Can you work these out from the model? Positions are in its coordinate system, mm. A direction names the side the tool comes from. Give positions to 0.01 mm unless a question says otherwise; leave off trailing zeros. Loops run counter-clockwise (first coordinate to the right, second up) from the corner with the lowest first, then second, coordinate; pieces in that order, holes last. Notation, with made-up numbers: (13.5, 30.25) - (50.5, 30.25) arc R23 ccw to (50.5, 63.25) - close; hole circle Ø5 at (0, -11). An arc over 180 degrees is marked (long way). Answer as a JSON object with one key per item and string values.
```python
from build123d import *

# Parameters (mm, degrees)
SKETCH1_R           = 17.5
SKETCH1_R_2         = 15
BOSS_EXTRUDE1_DEPTH = 10
SKETCH2_R           = 37.5
SKETCH2_R_2         = 27.5
BOSS_EXTRUDE2_DEPTH = 10


with BuildPart() as part:
    # Sketch1 → Boss-Extrude1 (new body)
    with BuildSketch(Plane(origin=(0, 0, 0), x_dir=(0, 0, -1), z_dir=(1, 0, 0))):
        with BuildLine():
            ThreePointArc((30.555677848, -21.739377894), (0, 37.5), (-30.555677848, -21.739377894))
            ThreePointArc((-30.555677848, -21.739377894), (-10, -78.973363491), (-22.221723794, -138.545961778))
            ThreePointArc((-22.221723794, -138.545961778), (0, -175), (22.221723794, -138.545961778))
            ThreePointArc((22.221723794, -138.545961778), (10, -78.973363491), (30.555677848, -21.739377894))
        make_face()
        Circle(SKETCH1_R, mode=Mode.SUBTRACT)
        with Locations((0, -150)):
            Circle(SKETCH1_R_2, mode=Mode.SUBTRACT)
    extrude(amount=BOSS_EXTRUDE1_DEPTH)

    # Sketch2 → Boss-Extrude2 (add)
    with BuildSketch(Plane.ZY):
        Circle(SKETCH2_R)
        Circle(SKETCH2_R_2, mode=Mode.SUBTRACT)
    extrude(amount=BOSS_EXTRUDE2_DEPTH)


solid = part.part
```
1) Imagine slicing it at C-C on y = -150. Write out the boundary of the cut face in (x, z), and give its area (3 significant figures).
Check sheet entries:
{"outline": "(0, -25) - (10, -25) - (10, -15) - (0, -15) - close; (0, 15) - (10, 15) - (10, 25) - (0, 25) - close", "area": "200 mm2"}
2) Imagine slicing it at D-D on x = 6.5. Write out the boundary of the cut face in (y, z).
Check sheet entries:
{"outline": "(-138.55, -22.22) arc R112.54 cw to (-21.74, -30.56) arc R37.5 ccw (long way) to (-21.74, 30.56) arc R112.54 cw to (-138.55, 22.22) arc R25 ccw (long way) to start; hole circle Ø30 at (-150, 0); hole circle Ø35 at (0, 0)"}
3) Which directions (+Z, -Z, +X, -X, +Y, -Y) give clear straight access to the entire face, cutting with the end or side of a thin tool? Please do faces 5 (the cylindrical face through (-4.93, -26.846, -5.961)), 6 (the cylindrical face through (4.93, -79.834, -9.942)).
Check sheet entries:
{"face 5": "-X", "face 6": "-Z, +X, -X"}
4) Imagine slicing it at A-A on y = 0. Write out the boundary of the cut face in (x, z).
Check sheet entries:
{"outline": "(-10, -37.5) - (10, -37.5) - (10, -17.5) - (0, -17.5) - (0, -27.5) - (-10, -27.5) - close; (-10, 27.5) - (0, 27.5) - (0, 17.5) - (10, 17.5) - (10, 37.5) - (-10, 37.5) - close"}
5) I'm going to push flat-ended pins straight in: P1, Ø6, axis at y = -64.5, z = -16.5, coming from the -X side; P2, Ø16.5, axis at y = 11.5, z = -3, coming from the -X side; P3, Ø4, axis at x = -4, z = 26.5, coming from the +Y side; P4, Ø6, axis at x = 4.5, y = -152, coming from the -Z side. Where does each tip first touch, or does it pass through?
Check sheet entries:
{"P1": "through", "P2": "x = 0", "P3": "y = 28.39", "P4": "z = -25"}
6) If we mould it in two halves opening along Z, with no side actions, what happens to faces 1 (the cylindrical face through (4.93, -78.114, 10.065)), 2 (the cylindrical face through (4.93, -163.31, -6.92)), 3 (the cylindrical face through (4.93, -174.99, 0.72)), 4 (the flat face through (-10, 20, -20))? For each: released by +Z, released by -Z, zero draft, split by the parting line, or undercut.
Check sheet entries:
{"face 1": "released by +Z", "face 2": "undercut", "face 3": "split by the parting line", "face 4": "zero draft"}
7) I need wall thicknesses on L1, parallel to Y at x = 5.25, z = 0; L2, parallel to X at y = 18, z = 18; L3, parallel to Y at x = -2.75, z = 0. Which ranges of each line are inside material? Lowest first, please.
Check sheet entries:
{"L1": "-175 to -165, -135 to -17.5, 17.5 to 37.5", "L2": "0 to 10", "L3": "-37.5 to -27.5, 27.5 to 37.5"}
8) Imagine slicing it at B-B on z = 0. Write out the boundary of the cut face in (x, y).
Check sheet entries:
{"outline": "(-10, -37.5) - (0, -37.5) - (0, -135) - (10, -135) - (10, -17.5) - (0, -17.5) - (0, -27.5) - (-10, -27.5) - close; (-10, 27.5) - (0, 27.5) - (0, 17.5) - (10, 17.5) - (10, 37.5) - (-10, 37.5) - close; (0, -175) - (10, -175) - (10, -165) - (0, -165) - close"}
